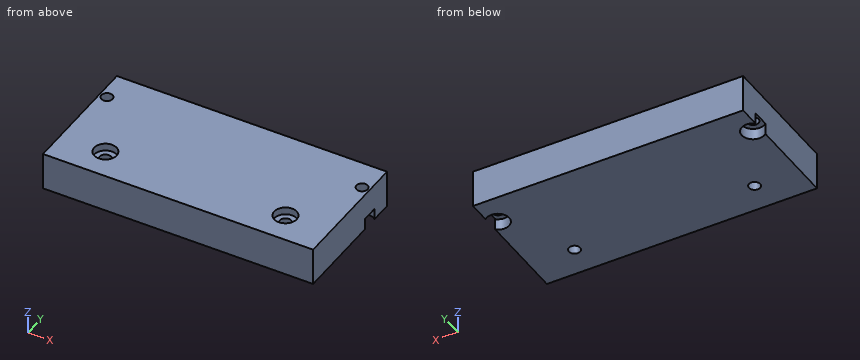
```python
from build123d import *

# Parameters (mm, degrees)
CYLINDER320_R     = 1.5
CYLINDER320_DEPTH = 50
CYLINDER321_R     = 1.5
CYLINDER321_DEPTH = 50
CYLINDER322_R     = 1.5
CYLINDER322_DEPTH = 50
CYLINDER319_R     = 1.5
CYLINDER319_DEPTH = 50
CYLINDER323_R     = 3
CYLINDER323_DEPTH = 4
CYLINDER325_R     = 3
CYLINDER325_DEPTH = 4
CYLINDER326_R     = 3
CYLINDER326_DEPTH = 4
CYLINDER324_R     = 3
CYLINDER324_DEPTH = 4
CYLINDER293_R     = 1.5
CYLINDER293_DEPTH = 50
CYLINDER294_R     = 1.5
CYLINDER294_DEPTH = 50
CYLINDER297_R     = 3
CYLINDER297_DEPTH = 4
CYLINDER298_R     = 3
CYLINDER298_DEPTH = 4
BOX138_W          = 72
BOX138_H          = 34
BOX138_DEPTH      = 10


with BuildPart() as obj1:
    # Cylinder320 → Cylinder320 (new body)
    with BuildSketch(Plane(origin=(-51, 6, 0), x_dir=(1, 0, 0), z_dir=(0, 0, 1))):
        Circle(CYLINDER320_R)
    extrude(amount=CYLINDER320_DEPTH)


with BuildPart() as obj2:
    # Cylinder321 → Cylinder321 (new body)
    with BuildSketch(Plane(origin=(-24, 18, 0), x_dir=(1, 0, 0), z_dir=(0, 0, 1))):
        Circle(CYLINDER321_R)
    extrude(amount=CYLINDER321_DEPTH)


with BuildPart() as obj3:
    # Cylinder322 → Cylinder322 (new body)
    with BuildSketch(Plane(origin=(24, 18, 0), x_dir=(1, 0, 0), z_dir=(0, 0, 1))):
        Circle(CYLINDER322_R)
    extrude(amount=CYLINDER322_DEPTH)


with BuildPart() as compound295:
    # Cylinder319 → Cylinder319 (new body)
    with BuildSketch(Plane(origin=(51, 6, 0), x_dir=(1, 0, 0), z_dir=(0, 0, 1))):
        Circle(CYLINDER319_R)
    extrude(amount=CYLINDER319_DEPTH)

    # Compound295: union obj1, obj2, obj3
    add(obj1.part)
    add(obj2.part)
    add(obj3.part)


with BuildPart() as obj4:
    # Cylinder323 → Cylinder323 (new body)
    with BuildSketch(Plane(origin=(-51, 7, 0), x_dir=(1, 0, 0), z_dir=(0, 0, 1))):
        Circle(CYLINDER323_R)
    extrude(amount=CYLINDER323_DEPTH)


with BuildPart() as obj5:
    # Cylinder325 → Cylinder325 (new body)
    with BuildSketch(Plane(origin=(-24, 18, 0), x_dir=(1, 0, 0), z_dir=(0, 0, 1))):
        Circle(CYLINDER325_R)
    extrude(amount=CYLINDER325_DEPTH)


with BuildPart() as obj6:
    # Cylinder326 → Cylinder326 (new body)
    with BuildSketch(Plane(origin=(24, 18, 0), x_dir=(1, 0, 0), z_dir=(0, 0, 1))):
        Circle(CYLINDER326_R)
    extrude(amount=CYLINDER326_DEPTH)


with BuildPart() as compound296:
    # Cylinder324 → Cylinder324 (new body)
    with BuildSketch(Plane(origin=(51, 7, 0), x_dir=(1, 0, 0), z_dir=(0, 0, 1))):
        Circle(CYLINDER324_R)
    extrude(amount=CYLINDER324_DEPTH)

    # Compound296: union obj4, obj5, obj6
    add(obj4.part)
    add(obj5.part)
    add(obj6.part)


with BuildPart() as compound296_1:
    # Compound296 placement: moved
    add(compound296.part.moved(Location((0, 0, 8))))


with BuildPart() as obj7:
    # Cylinder293 → Cylinder293 (new body)
    with BuildSketch(Plane(origin=(34, 36, 0), x_dir=(1, 0, 0), z_dir=(0, 0, 1))):
        Circle(CYLINDER293_R)
    extrude(amount=CYLINDER293_DEPTH)


with BuildPart() as compound284:
    # Cylinder294 → Cylinder294 (new body)
    with BuildSketch(Plane(origin=(-34, 36, 0), x_dir=(1, 0, 0), z_dir=(0, 0, 1))):
        Circle(CYLINDER294_R)
    extrude(amount=CYLINDER294_DEPTH)

    # Compound284: union obj7
    add(obj7.part)


with BuildPart() as obj8:
    # Cylinder297 → Cylinder297 (new body)
    with BuildSketch(Plane(origin=(34, 36, -1), x_dir=(1, 0, 0), z_dir=(0, 0, 1))):
        Circle(CYLINDER297_R)
    extrude(amount=CYLINDER297_DEPTH)


with BuildPart() as compound282:
    # Cylinder298 → Cylinder298 (new body)
    with BuildSketch(Plane(origin=(-34, 36, -1), x_dir=(1, 0, 0), z_dir=(0, 0, 1))):
        Circle(CYLINDER298_R)
    extrude(amount=CYLINDER298_DEPTH)

    # Compound282: union obj8
    add(obj8.part)


with BuildPart() as cut141:
    # Box138 → Box138 (new body)
    with BuildSketch(Plane(origin=(-36, 10, 0), x_dir=(1, 0, 0), z_dir=(0, 0, 1))):
        with Locations((36, 17)):
            Rectangle(BOX138_W, BOX138_H)
    extrude(amount=BOX138_DEPTH)

    # Cut131: cut Compound282
    add(compound282.part, mode=Mode.SUBTRACT)

    # Cut132: cut Compound284
    add(compound284.part, mode=Mode.SUBTRACT)

    # Cut140: cut Compound296
    add(compound296_1.part, mode=Mode.SUBTRACT)

    # Cut141: cut Compound295
    add(compound295.part, mode=Mode.SUBTRACT)


solid = cut141.part
```
Verification items for the finished model (mm, model axes). Round coordinates to 2 decimals unless told otherwise and drop trailing zeros. Write each loop counter-clockwise with the first axis right and the second up, starting at its lowest first coordinate (ties: lowest second). Pieces come first, ordered by that corner, then holes.
1. Section check B-B on y = 18. Enter the section's corners in (x, z).
2. Section check A-A on x = -24. Enter the section's corners in (y, z).
3. Scan lines: L1, parallel to X at y = 18, z = 9.45; L2, parallel to X at y = 36, z = 7.5; L3, parallel to Y at x = 34, z = 1.5. Record each from-to range of solid material in increasing order.
4. Gauge pin test, flat ends, axial feed: P1, Ø3.5, axis at x = -24, y = 18, coming from the +Z side; P2, Ø2.5, axis at x = -34.5, y = 37.5, coming from the -Z side; P3, Ø2.5, axis at x = -24, y = 18, coming from the +Z side. Record the tip position at first contact, or that the pin passes through.
5. Section check C-C on x = -34. Enter the section's corners in (y, z).
Answer:
1. outline: (-36, 0) - (-25.5, 0) - (-25.5, 8) - (-27, 8) - (-27, 10) - (-36, 10) - close; (-22.5, 0) - (22.5, 0) - (22.5, 8) - (21, 8) - (21, 10) - (-21, 10) - (-21, 8) - (-22.5, 8) - close; (25.5, 0) - (36, 0) - (36, 10) - (27, 10) - (27, 8) - (25.5, 8) - close
2. outline: (10, 0) - (16.5, 0) - (16.5, 8) - (15, 8) - (15, 10) - (10, 10) - close; (19.5, 0) - (44, 0) - (44, 10) - (21, 10) - (21, 8) - (19.5, 8) - close
3. L1: x = -36 to -27, -21 to 21, 27 to 36
3. L2: x = -36 to -35.5, -32.5 to 32.5, 35.5 to 36
3. L3: y = 10 to 33, 39 to 44
4. P1: stops at z = 8
4. P2: stops at z = 3
4. P3: passes through
5. outline: (10, 0) - (33, 0) - (33, 3) - (34.5, 3) - (34.5, 10) - (10, 10) - close; (37.5, 3) - (39, 3) - (39, 0) - (44, 0) - (44, 10) - (37.5, 10) - close
